Input: part model. Units: mm. Frame: model coordinates. Give positions to 0.01 mm unless a question says otherwise; leave off trailing zeros. Write each loop counter-clockwise with the first axis right and the second up, starting at its lowest first coordinate (ties: lowest second). Pieces come first, ordered by that corner, then holes. Notation, with made-up numbers: (37.25, -9) -> (63.25, -9) arc R14 ccw to (63.25, -4) -> close; hole circle Ø9 at (89, 82.5). An arc over 180 degrees is marked (long way). Return JSON: item names as keys, results as strings. Group by question number.
Item 1: Section B-B, the plane z = 37.5. Return loops of the section in (x, y).
Item 2: Line query: line 1 (X direction, y = 1.7, z = -42.94); line 2 (X direction, y = 1.3, z = -20); line 3 (Z direction, x = -11.5, y = 1.65). Output: solid intervals per line, ascending. Write a range as [from, to].
Item 3: Section C-C, the plane x = 0. Return loops of the section in (y, z), then the cut area to 3 significant figures.
Item 4: Section D-D, the plane z = 0. Return loops of the section in (x, y).
Item 5: Section A-A, the plane x = 10. Return loops of the section in (y, z), then the cut area to 3 significant figures.
Item 6: Pin query (flat end, axial travel): P1, Ø3.5, axis at x = -22, z = -42.94, coming from the -Y side; P2, Ø1.5, axis at y = 2, z = -5, coming from the +X side; P3, Ø1, axis at x = -8, y = 1.5, coming from the +Z side. Return the tip coordinate at first contact, or that it passes through.
from build123d import *

# Parameters (mm, degrees)
SKETCH1_R           = 1.609204822
SKETCH1_R_2         = 2.3
SKETCH1_R_3         = 3.5
BOSS_EXTRUDE1_DEPTH = 3


with BuildPart() as part:
    # Sketch1 → Boss-Extrude1 (new body)
    with BuildSketch(Plane(origin=(0, 0, 0), x_dir=(1, 0, 0), z_dir=(0, 1, 0))):
        Polygon((-30.75, 58.5), (-30.75, 19.5), (-27.75, 19.5), (-27.75, -19.5), (-30.75, -19.5), (-30.75, -58.5), (-14, -58.5), (-14, -55.5), (14, -55.5), (14, -58.5), (30.75, -58.5), (30.75, -19.5), (27.75, -19.5), (27.75, 19.5), (30.75, 19.5), (30.75, 58.5), (14, 58.5), (14, 55.5), (-14, 55.5), (-14, 58.5), align=None)
        with Locations(Location((-22, -42.94, 0), (0, 0, 270))):
            Circle(SKETCH1_R, mode=Mode.SUBTRACT)
        with Locations(Location((22, -42.94, 0), (0, 0, 270))):
            Circle(SKETCH1_R, mode=Mode.SUBTRACT)
        with Locations(Location((22, 42.94, 0), (0, 0, 270))):
            Circle(SKETCH1_R, mode=Mode.SUBTRACT)
        with Locations(Location((-22, 42.94, 0), (0, 0, 270))):
            Circle(SKETCH1_R, mode=Mode.SUBTRACT)
        with Locations(Location((0, 37.5, 0), (0, 0, 270))):
            Circle(SKETCH1_R_2, mode=Mode.SUBTRACT)
        with Locations(Location((0, -37.5, 0), (0, 0, 270))):
            Circle(SKETCH1_R_2, mode=Mode.SUBTRACT)
        with Locations(Location((-10, -20, 0), (0, 0, 270))):
            Circle(SKETCH1_R_3, mode=Mode.SUBTRACT)
        with Locations(Location((10, -20, 0), (0, 0, 270))):
            Circle(SKETCH1_R_3, mode=Mode.SUBTRACT)
        with Locations(Location((-10, 0, 0), (0, 0, 270))):
            Circle(SKETCH1_R_3, mode=Mode.SUBTRACT)
        with Locations(Location((10, 0, 0), (0, 0, 270))):
            Circle(SKETCH1_R_3, mode=Mode.SUBTRACT)
        with Locations(Location((-10, 20, 0), (0, 0, 270))):
            Circle(SKETCH1_R_3, mode=Mode.SUBTRACT)
        with Locations(Location((10, 20, 0), (0, 0, 270))):
            Circle(SKETCH1_R_3, mode=Mode.SUBTRACT)
    extrude(amount=BOSS_EXTRUDE1_DEPTH)


solid = part.part
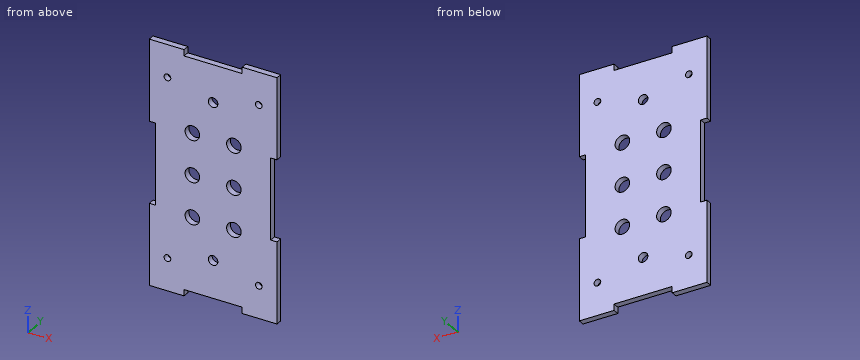
Answer below:
{
 "1": {"outline": "(-30.75, 0) -> (-2.3, 0) -> (-2.3, 3) -> (-30.75, 3) -> close; (2.3, 0) -> (30.75, 0) -> (30.75, 3) -> (2.3, 3) -> close"},
 "2": {"line 1": "x = [-30.75, -23.61], [-20.39, 20.39], [23.61, 30.75]", "line 2": "x = [-30.75, -13.5], [-6.5, 6.5], [13.5, 30.75]", "line 3": "z = [-55.5, -23.16], [-16.84, -3.16], [3.16, 16.84], [23.16, 55.5]"},
 "3": {"outline": "(0, -55.5) -> (3, -55.5) -> (3, -39.8) -> (0, -39.8) -> close; (0, -35.2) -> (3, -35.2) -> (3, 35.2) -> (0, 35.2) -> close; (0, 39.8) -> (3, 39.8) -> (3, 55.5) -> (0, 55.5) -> close", "area": "305 mm2"},
 "4": {"outline": "(-27.75, 0) -> (-13.5, 0) -> (-13.5, 3) -> (-27.75, 3) -> close; (-6.5, 0) -> (6.5, 0) -> (6.5, 3) -> (-6.5, 3) -> close; (13.5, 0) -> (27.75, 0) -> (27.75, 3) -> (13.5, 3) -> close"},
 "5": {"outline": "(0, -55.5) -> (3, -55.5) -> (3, -23.5) -> (0, -23.5) -> close; (0, -16.5) -> (3, -16.5) -> (3, -3.5) -> (0, -3.5) -> close; (0, 3.5) -> (3, 3.5) -> (3, 16.5) -> (0, 16.5) -> close; (0, 23.5) -> (3, 23.5) -> (3, 55.5) -> (0, 55.5) -> close", "area": "270 mm2"},
 "6": {"P1": "stops at y = 0", "P2": "stops at x = 27.75", "P3": "stops at z = 55.5"}
}
